Check sheet for the modelled part. Datum: model origin and axes. Units: mm. A direction names the side the tool comes from. Round coordinates to 2 decimals unless told otherwise and drop trailing zeros. Order: outer loops, then holes, each group sorted by start corner. A loop starts at its lowest first (then second) coordinate and runs counter-clockwise, first axis right, second up.
from build123d import *

# Parameters (mm, degrees)
F0_W     = 101.6
F0_H     = 44.45
F1_DEPTH = 25.4
F2_R     = 10.16
F4_DEPTH = 101.6
F6_DEPTH = 25.4
F8_DEPTH = 38.1


with BuildPart() as f1:
    # F0 (on Front) → F1 (new body)
    with BuildSketch(Plane.XZ):
        with Locations((-50.8, -22.225)):
            Rectangle(F0_W, F0_H)
    extrude(amount=F1_DEPTH)

    # F2
    f2_edges = [f1.edges().sort_by_distance(p)[0] for p in [
        (-50.8, -25.4, 0),
        (0, -12.7, 0),
        (0, -25.4, -22.225),
        (0, 0, -22.225),
        (-101.6, -25.4, -22.225),
        (-101.6, -12.7, 0),
        (-50.8, 0, 0),
        (-101.6, 0, -22.225),
    ]]
    fillet(f2_edges, radius=F2_R)

    # F3 (on face) → F4 (cut)
    with BuildSketch(Plane(origin=(-101.6, 0, 0), x_dir=(0, -1, 0), z_dir=(-1, 0, 0))):
        Polygon((15.24, -10.16), (10.16, -10.16), (10.16, -38.1), (12.7, -38.1), (15.24, -38.1), align=None)
    extrude(amount=-F4_DEPTH, mode=Mode.SUBTRACT)

    # F5 (on face) → F6 (cut)
    with BuildSketch(Plane.XZ.offset(25.4)):
        with BuildLine():
            Line((-77.47, -27.305), (-71.12, -27.305))
            ThreePointArc((-71.12, -27.305), (-72.979872, -22.814872), (-77.47, -20.955))
            Line((-77.47, -20.955), (-77.47, -27.305))
        make_face()
        with BuildLine():
            ThreePointArc((-17.78, -27.305), (-24.13, -20.955), (-30.48, -27.305))
            Line((-30.48, -27.305), (-24.13, -27.305))
            Line((-24.13, -27.305), (-17.78, -27.305))
        make_face()
        with BuildLine():
            Line((-24.13, -27.305), (-30.48, -27.305))
            ThreePointArc((-30.48, -27.305), (-24.13, -33.655), (-17.78, -27.305))
            Line((-17.78, -27.305), (-24.13, -27.305))
        make_face()
        with BuildLine():
            ThreePointArc((-44.45, -27.305), (-50.8, -20.955), (-57.15, -27.305))
            Line((-57.15, -27.305), (-50.8, -27.305))
            Line((-50.8, -27.305), (-44.45, -27.305))
        make_face()
        with BuildLine():
            Line((-50.8, -27.305), (-57.15, -27.305))
            ThreePointArc((-57.15, -27.305), (-50.8, -33.655), (-44.45, -27.305))
            Line((-44.45, -27.305), (-50.8, -27.305))
        make_face()
        with BuildLine():
            ThreePointArc((-77.47, -33.655), (-72.979872, -31.795128), (-71.12, -27.305))
            Line((-71.12, -27.305), (-77.47, -27.305))
            Line((-77.47, -27.305), (-77.47, -33.655))
        make_face()
        with BuildLine():
            Line((-77.47, -27.305), (-77.47, -20.955))
            ThreePointArc((-77.47, -20.955), (-81.960128, -22.814872), (-83.82, -27.305))
            Line((-83.82, -27.305), (-77.47, -27.305))
        make_face()
        with BuildLine():
            ThreePointArc((-83.82, -27.305), (-81.960128, -31.795128), (-77.47, -33.655))
            Line((-77.47, -33.655), (-77.47, -27.305))
            Line((-77.47, -27.305), (-83.82, -27.305))
        make_face()
    extrude(amount=-F6_DEPTH, mode=Mode.SUBTRACT)

    # F7 (on face) → F8 (cut)
    with BuildSketch(Plane.XY):
        Polygon((-50.8, -8.89), (-82.55, -8.89), (-82.55, -12.7), (-82.55, -16.51), (-50.8, -16.51), (-19.05, -16.51), (-19.05, -12.7), (-19.05, -8.89), align=None)
    extrude(amount=-F8_DEPTH, mode=Mode.SUBTRACT)


solid = f1.part
1) Sectioned sample at B-B on x = -50.8. Record the cut outline in (y, z) (3 decimals), and give its area (3 significant figures).
2) Sectioned sample at A-A on x = -88. Record the cut outline in (y, z), and give its area (3 significant figures).
3) Sectioned sample at D-D on x = -64. Record the cut outline in (y, z).
4) Gauge pin test, flat ends, axial feed: pin 1 (2.5 mm diameter, centred on x = -58.5, y = -11, fed in from +Z); pin 2 (1 mm diameter, centred on y = -16, z = -34.5, fed in from +X); pin 3 (10 mm diameter, centred on x = -24.13, z = -27.305, fed in from +Y); pin 4 (6 mm diameter, centred on x = -18.5, y = -22, fed in from +Z). Record the tip position at first contact, or that the pin passes through.
5) Scan lines: line 1 (X direction, y = -20.25, z = -27); line 2 (Y direction, x = -52.5, z = -36); line 3 (Z direction, x = -14.5, y = -11). Record each from-to range of solid material in increasing order.
6) Set-up check for faces 1 (the face through (-15, -13, 0)), 2 (the face through (-10, -10.16, -24)), 3 (the face through (-50.231, -3.055, -2.897)), 4 (the face through (-82.55, -13, -9)), 5 (the face through (-52, -13, -38.1)): record each of +Z, -Z, +X, -X, +Y, -Y from which the full face is reachable in a straight line by a thin tool's end or side.
7) Sectioned sample at C-C on y = -2.25. Record the cut outline in (x, z) (3 decimals).
8) Draft check along X on faces 6 (the face through (-98.703, -3.055, -27.065)), 7 (the face through (-92, -10.16, -24)), 8 (the face through (-17.786, -20.391, -27.584)). Enter one of: pulls with the +X half, pulls with the -X half, needs draft (parallel to the pull), parting line crosses it, or undercut.
Values found:
1. outline: (-25.4, -44.45) - (0, -44.45) - (0, -33.655) - (-8.89, -33.655) - (-8.89, -38.1) - (-16.51, -38.1) - (-16.51, -33.655) - (-25.4, -33.655) - close; (-25.4, -20.955) - (-16.51, -20.955) - (-16.51, -0.08) arc R10.16 ccw to (-25.4, -10.16) - close; (-8.89, -20.955) - (0, -20.955) - (0, -10.16) arc R10.16 ccw to (-8.89, -0.08) - close
1. area: 569 mm2
2. outline: (-25.4, -44.45) - (0, -44.45) - (0, -10.16) arc R10.16 ccw to (-10.16, 0) - (-15.24, 0) arc R10.16 ccw to (-25.4, -10.16) - close; hole (-15.24, -38.1) - (-10.16, -38.1) - (-10.16, -10.16) - (-15.24, -10.16) - close
2. area: 943 mm2
3. outline: (-25.4, -44.45) - (0, -44.45) - (0, -10.16) arc R10.16 ccw to (-8.89, -0.08) - (-8.89, -38.1) - (-16.51, -38.1) - (-16.51, -0.08) arc R10.16 ccw to (-25.4, -10.16) - close
4. pin 1: stops at z = -38.1
4. pin 2: stops at x = 0
4. pin 3: passes through
4. pin 4: stops at z = -0.72
5. line 1: x = -100.28 to -83.81, -71.13 to -57.14, -44.46 to -30.47, -17.79 to -1.32
5. line 2: y = -25.4 to -16.51, -8.89 to 0
5. line 3: z = -44.45 to -38.1, -10.16 to 0
6. face 1: +Z, +X, -X, +Y, -Y
6. face 2: +X, -X
6. face 3: +Z, +X, -X, +Y
6. face 4: +Z
6. face 5: none
7. outline: (-97.816, -44.45) - (-3.784, -44.45) - (-3.784, -10.16) arc R6.376 ccw to (-10.16, -3.784) - (-91.44, -3.784) arc R6.376 ccw to (-97.816, -10.16) - close; hole circle Ø12.7 at (-77.47, -27.305); hole circle Ø12.7 at (-50.8, -27.305); hole circle Ø12.7 at (-24.13, -27.305)
8. face 6: pulls with the -X half
8. face 7: needs draft
8. face 8: undercut
